Check sheet for the modelled part. Datum: model origin and axes. Units: mm. Face numbers are marked on the shaded views. A direction names the side the tool comes from. Coordinates: 2 decimals unless noted, no trailing zeros. Write each loop counter-clockwise with the first axis right and the second up, starting at its lowest first coordinate (ties: lowest second). Pieces come first, ordered by that corner, then holes. Notation, with made-up numbers: (38.5, 6.25) - (69.5, 6.25) arc R24 ccw to (69.5, 38.25) - close; hole circle Ø10 at (59.5, 51). An arc over 180 degrees is marked (long way). Write each question's results on one line, items separated by ' | '.
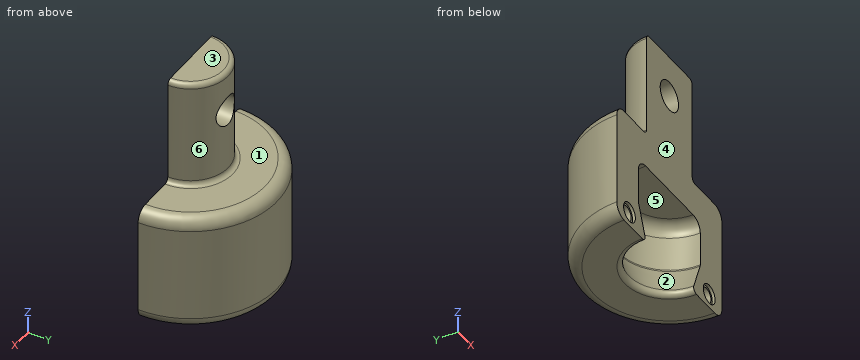
from build123d import *

# Parameters (mm, degrees)
F1_ANGLE = -180
F2_R     = 2
F3_R     = 4.1
F3_R_2   = 3.2
F4_DEPTH = 1.2
F5_DEPTH = 12
F3_R_3   = 6.35
F6_DEPTH = 36.460554
F7_R     = 5


with BuildPart() as f1:
    # F0 (on Front) → F1 (revolve)
    with BuildSketch(Plane.XZ):
        with BuildLine():
            Line((21.459554, 35), (21.459554, 15))
            Line((21.459554, 15), (21.459554, 0))
            Line((21.459554, 0), (36.459554, 0))
            Line((36.459554, 0), (36.459554, 50))
            Line((36.459554, 50), (15.8496, 50))
            Line((15.8496, 50), (15.8496, 96.101))
            Line((15.8496, 96.101), (0, 96.101))
            Line((0, 96.101), (0, 84.671))
            ThreePointArc((0, 84.671), (4.490128, 82.811128), (6.35, 78.321))
            ThreePointArc((6.35, 78.321), (4.490128, 73.830872), (0, 71.971))
            Line((0, 71.971), (0, 35))
            Line((0, 35), (21.459554, 35))
        make_face()
        Polygon((21.459554, 15), (16, 0), (21.459554, 0), align=None)
    revolve(axis=Axis((0, 0, 65.5505), (0, 0, -1)), revolution_arc=F1_ANGLE)

    # F2
    f2_edges = [f1.edges().sort_by_distance(p)[0] for p in [
        (0, 15.8496, 50),
        (0, 15.8496, 96.101),
        (0, 16, 0),
        (0, 21.459554, 15),
    ]]
    fillet(f2_edges, radius=F2_R)

    # F3 (on Front) → F4 (cut)
    with BuildSketch(Plane.XZ):
        with Locations((27.657925, 6.15)):
            Circle(F3_R)
        with Locations((27.657925, 6.15)):
            Circle(F3_R_2, mode=Mode.SUBTRACT)
        with Locations((-27.657925, 6.15)):
            Circle(F3_R)
        with Locations((-27.657925, 6.15)):
            Circle(F3_R_2, mode=Mode.SUBTRACT)
        with Locations((-27.657925, 6.15)):
            Circle(F3_R_2)
        with Locations((27.657925, 6.15)):
            Circle(F3_R_2)
    extrude(amount=-F4_DEPTH, mode=Mode.SUBTRACT)

    # F3 (on Front) → F5 (cut)
    with BuildSketch(Plane.XZ):
        with Locations((-27.657925, 6.15)):
            Circle(F3_R_2)
        with Locations((27.657925, 6.15)):
            Circle(F3_R_2)
    extrude(amount=-F5_DEPTH, mode=Mode.SUBTRACT)

    # F3 (on Front) → F6 (cut, through all)
    with BuildSketch(Plane.XZ):
        with Locations((0, 78.321)):
            Circle(F3_R_3)
    extrude(amount=-F6_DEPTH, mode=Mode.SUBTRACT)

    # F7
    f7_edges = [f1.edges().sort_by_distance(p)[0] for p in [
        (0, 36.459554, 50),
        (0, 36.459554, 0),
        (0, 21.459554, 35),
    ]]
    fillet(f7_edges, radius=F7_R)


solid = f1.part
1. Sectioned sample at C-C (z = 90.5). Record the cut outline in (x, y).
Values follow:
outline: (-15.85, 0) - (15.85, 0) arc R15.85 ccw to start
2. Go/stop test with flat-tipped pins: pin 1 (10.5 mm diameter, centred on x = 27.66, z = 6.15, fed in from +Y); pin 2 (5 mm diameter, centred on y = 16, z = 67, fed in from -X); pin 3 (8 mm diameter, centred on x = -8, y = 28, fed in from +Z). Record where each tip stops, or that it passes through.
Values follow:
pin 1: stops at y = 28.76 | pin 2: stops at x = -8.3 | pin 3: stops at z = 50
3. Sectioned sample at A-A (z = 6.15). Record the cut outline in (x, y), then the cut area to 3 significant figures.
Values follow:
outline: (-36.46, 0) - (-31.76, 0) - (-31.76, 1.2) - (-30.86, 1.2) - (-30.86, 12) - (-24.46, 12) - (-24.46, 1.2) - (-23.56, 1.2) - (-23.56, 0) - (-18.24, 0) arc R18.24 cw to (18.24, 0) - (23.56, 0) - (23.56, 1.2) - (24.46, 1.2) - (24.46, 12) - (30.86, 12) - (30.86, 1.2) - (31.76, 1.2) - (31.76, 0) - (36.46, 0) arc R36.46 ccw to start | area: 1,410 mm^2
4. Draft check along X on the marked faces 4, 5 and 6. Enter one of: pulls with the +X half, pulls with the -X half, needs draft (parallel to the pull), parting line crosses it, or undercut.
Values follow:
face 4: needs draft | face 5: undercut | face 6: parting line crosses it
5. Material ranges on L1, parallel to Z at x = 0, y = 7; L2, parallel to Z at x = 27, y = 10; L3, parallel to Z at x = -1, y = 30, recorded low to high. Write a range as [from, to].
Values follow:
L1: z = [35, 71.97], [84.67, 96.1] | L2: z = [0, 3.02], [9.28, 50] | L3: z = [0, 50]
6. Sectioned sample at B-B (z = 20). Record the cut outline in (x, y), then the cut area to 3 significant figures.
Values follow:
outline: (-36.46, 0) - (-21.46, 0) arc R21.46 cw to (21.46, 0) - (36.46, 0) arc R36.46 ccw to start | area: 1,360 mm^2
7. Access from +Z, -Z, +X, -X, +Y, -Y to the whole of each face (thin tool, end or side, straight path). Record for the marked faces 1, 2 and 3.
Values follow:
face 1: +Z, +Y | face 2: -Y | face 3: +Z, +X, -X, +Y, -Y
